Geometry check sheet. Reference: the model listing, model coordinates, mm. Round coordinates to 2 decimals unless told otherwise and drop trailing zeros. Loops run counter-clockwise (first coordinate to the right, second up) from the corner with the lowest first, then second, coordinate; pieces in that order, holes last.
```python
from build123d import *

# Parameters (mm, degrees)
SKETCH4_R           = 1
SKETCH4_R_2         = 0.75
BOSS_EXTRUDE1_DEPTH = 1.6


with BuildPart() as part:
    # Sketch4 → Boss-Extrude1 (new body)
    with BuildSketch(Plane.XY):
        Polygon((0, 40), (-32, 40), (-32, 20), (-15, 16), (-15, 6), (-11, 6), (-11, 0), (0, 0), align=None)
        with Locations((-30, 26)):
            Circle(SKETCH4_R, mode=Mode.SUBTRACT)
        with Locations((-8.7, 9.7)):
            Circle(SKETCH4_R_2, mode=Mode.SUBTRACT)
    boss_extrude1 = extrude(amount=BOSS_EXTRUDE1_DEPTH)

    # Mirror1: Boss-Extrude1 across plane
    add(boss_extrude1.mirror(Plane(origin=(0, 0, 1.6), x_dir=(0, 0, 1), z_dir=(-1, 0, 0))))


solid = part.part
```
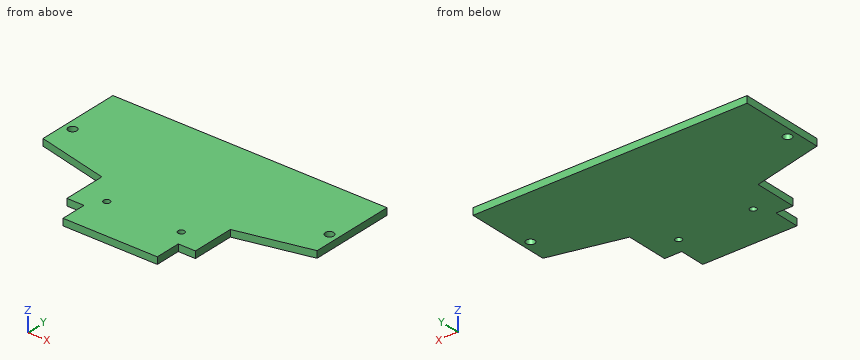
1) Scan lines: line 1 along Y through (x, z) = (8.7, 0.4); line 2 along Y through (x, z) = (30, 0.5); line 3 along Y through (x, z) = (-25.5, 0.35). Record each from-to range of solid material in increasing order.
Report:
line 1: y = 0 to 8.95, 10.45 to 40
line 2: y = 19.53 to 25, 27 to 40
line 3: y = 18.47 to 40
2) Sectioned sample at B-B, the plane y = 9.7. Record the cut outline in (x, z), then the cut area to 3 significant figures.
Report:
outline: (-15, 0) - (-9.45, 0) - (-9.45, 1.6) - (-15, 1.6) - close; (-7.95, 0) - (7.95, 0) - (7.95, 1.6) - (-7.95, 1.6) - close; (9.45, 0) - (15, 0) - (15, 1.6) - (9.45, 1.6) - close
area: 43.2 mm2
3) Gauge pin test, flat ends, axial feed: pin 1 (0.5 mm diameter, centred on y = 2, z = 0.5, fed in from -X); pin 2 (0.8 mm diameter, centred on y = 9, z = 1, fed in from -X). Record the tip position at first contact, or that the pin passes through.
Report:
pin 1: stops at x = -11
pin 2: stops at x = -15
4) Sectioned sample at A-A, the plane x = 8.7. Record the cut outline in (y, z), then the cut area to 3 significant figures.
Report:
outline: (0, 0) - (8.95, 0) - (8.95, 1.6) - (0, 1.6) - close; (10.45, 0) - (40, 0) - (40, 1.6) - (10.45, 1.6) - close
area: 61.6 mm2
5) Sectioned sample at D-D, the plane x = -30. Record the cut outline in (y, z).
Report:
outline: (19.53, 0) - (25, 0) - (25, 1.6) - (19.53, 1.6) - close; (27, 0) - (40, 0) - (40, 1.6) - (27, 1.6) - close
6) Sectioned sample at C-C, the plane z = 0.6. Record the cut outline in (x, y).
Report:
outline: (-32, 20) - (-15, 16) - (-15, 6) - (-11, 6) - (-11, 0) - (11, 0) - (11, 6) - (15, 6) - (15, 16) - (32, 20) - (32, 40) - (-32, 40) - close; hole circle Ø2 at (-30, 26); hole circle Ø1.5 at (-8.7, 9.7); hole circle Ø1.5 at (8.7, 9.7); hole circle Ø2 at (30, 26)
